```python
from build123d import *

# Parameters (mm, degrees)
SKETCH_1_R          = 6.35
EXTRUDE_1_DEPTH     = 2
SKETCH_2_R          = 4.75
EXTRUDE_2_DEPTH     = 5
SKETCH_3_R          = 3.25
CUT_EXTRUDE_1_DEPTH = 12.386175829
SKETCH_4_R          = 9.5
EXTRUDE_3_DEPTH     = 25


with BuildPart() as part:
    # 草图1 → 凸台-拉伸1 (new body)
    with BuildSketch(Plane(origin=(0, 0, 0), x_dir=(1, 0, 0), z_dir=(0, 1, 0))):
        with Locations(Location((0, 0, 0), (0, 0, 270))):
            Circle(SKETCH_1_R)
    extrude(amount=EXTRUDE_1_DEPTH)

    # 草图2 → 凸台-拉伸2 (add)
    with BuildSketch(Plane(origin=(0, 2, 0), x_dir=(1, 0, 0), z_dir=(0, 1, 0))):
        with Locations(Location((0, 0, 0), (0, 0, 270))):
            Circle(SKETCH_2_R)
    extrude(amount=EXTRUDE_2_DEPTH)

    # 草图3 → 切除-拉伸1 (cut, through all)
    with BuildSketch(Plane(origin=(0, 7, 0), x_dir=(1, 0, 0), z_dir=(0, 1, 0))):
        with Locations(Location((0, 0, 0), (0, 0, 270))):
            Circle(SKETCH_3_R)
    extrude(amount=-CUT_EXTRUDE_1_DEPTH, mode=Mode.SUBTRACT)

    # 草图4 → 凸台-拉伸3 (add)
    with BuildSketch(Plane.XZ):
        with Locations(Location((0, 0, 0), (0, 0, 270))):
            Circle(SKETCH_4_R)
    extrude(amount=EXTRUDE_3_DEPTH)


solid = part.part
```
Geometry check sheet. Reference: the model listing, model coordinates, mm. A direction names the side the tool comes from. Give positions to 0.01 mm unless a question says otherwise; leave off trailing zeros. Write each loop counter-clockwise with the first axis right and the second up, starting at its lowest first coordinate (ties: lowest second). Pieces come first, ordered by that corner, then holes. Notation, with made-up numbers: (67.25, 56.5) -> (124.25, 56.5) arc R24 ccw to (124.25, 78.5) -> close; hole circle Ø7 at (85, 25.25). An arc over 180 degrees is marked (long way). Use one line per item in the form item = value.
Item 1: Access from +Z, -Z, +X, -X, +Y, -Y to the whole of each face (thin tool, end or side, straight path). Record for faces 4 (the cylindrical face through (-1.978, 3.549, -2.579)), 5 (the flat face through (0, -25, 0)).
Results list:
face_4 = +Y
face_5 = +Z, -Z, +X, -X, -Y
Item 2: Sectioned sample at C-C on y = -5.5. Enter the section's corners in (x, z), plus the area to 3 significant figures.
Results list:
outline = circle Ø19 at (0, 0)
area = 284 mm2
Item 3: Scan lines: line 1 (X direction, y = 3.5, z = 0); line 2 (Y direction, x = -6, z = -3.75); line 3 (Y direction, x = 4.75, z = -3.75). Record each from-to range of solid material in increasing order.
Results list:
line_1 = -4.75 to -3.25, 3.25 to 4.75
line_2 = -25 to 0
line_3 = -25 to 2
Item 4: Sectioned sample at B-B on x = 0. Enter the section's corners in (y, z), plus the area to 3 significant figures.
Results list:
outline = (-25, -9.5) -> (0, -9.5) -> (0, -6.35) -> (2, -6.35) -> (2, -4.75) -> (7, -4.75) -> (7, -3.25) -> (0, -3.25) -> (0, 3.25) -> (7, 3.25) -> (7, 4.75) -> (2, 4.75) -> (2, 6.35) -> (0, 6.35) -> (0, 9.5) -> (-25, 9.5) -> close
area = 502 mm2
Item 5: Mould release check, pull along Z, two halves, no side actions. Record for faces 1 (the flat face through (-5, 2, 1)), 2 (the flat face through (0, 0, 0)), 3 (the cylindrical face through (-3.86, 0.99, -5.04)): released by +Z, released by -Z, zero draft, split by the parting line, or undercut.
Results list:
face_1 = zero draft
face_2 = undercut
face_3 = split by the parting line
Item 6: Sectioned sample at D-D on x = -4. Enter the section's corners in (y, z).
Results list:
outline = (-25, -8.62) -> (0, -8.62) -> (0, -4.93) -> (2, -4.93) -> (2, -2.56) -> (7, -2.56) -> (7, 2.56) -> (2, 2.56) -> (2, 4.93) -> (0, 4.93) -> (0, 8.62) -> (-25, 8.62) -> close
Item 7: Depth check by flat-ended pin: pin 1 Ø1 at (x, z) = (-6, -7.5) entering from +Y; pin 2 Ø4 at (x, y) = (-5.5, -14) entering from -Z; pin 3 Ø1 at (y, z) = (-1, -5) entering from -X. Enter the tip coordinate at first touch or a pass-through.
Results list:
pin_1 = 0
pin_2 = -8.83
pin_3 = -8.37
Item 8: Sectioned sample at A-A on z = 0. Enter the section's corners in (x, y), plus the area to 3 significant figures.
Results list:
outline = (-9.5, -25) -> (9.5, -25) -> (9.5, 0) -> (6.35, 0) -> (6.35, 2) -> (4.75, 2) -> (4.75, 7) -> (3.25, 7) -> (3.25, 0) -> (-3.25, 0) -> (-3.25, 7) -> (-4.75, 7) -> (-4.75, 2) -> (-6.35, 2) -> (-6.35, 0) -> (-9.5, 0) -> close
area = 502 mm2
